```python
from build123d import *

# Parameters (mm, degrees)
F0_W     = 97.79
F0_H     = 57.15
F1_DEPTH = 14.7828
F2_W     = 38.1
F2_H     = 57.15
F3_DEPTH = 11.97483
F4_R     = 5
F6_DEPTH = 26.75863


with BuildPart() as f1:
    # F0 (on Front) → F1 (new body)
    with BuildSketch(Plane.XZ):
        with Locations((48.895, 28.575)):
            Rectangle(F0_W, F0_H)
    extrude(amount=F1_DEPTH)

    # F2 (on face) → F3 (join)
    with BuildSketch(Plane.XZ.offset(14.7828)):
        with Locations((48.895, 28.575)):
            Rectangle(F2_W, F2_H)
    extrude(amount=F3_DEPTH)

    # F4
    f4_edges = [f1.edges().sort_by_distance(p)[0] for p in [
        (0, -7.3914, 0),
        (29.845, -20.770215, 0),
        (67.945, -20.770215, 0),
        (97.79, -7.3914, 0),
        (97.79, -7.3914, 57.15),
        (67.945, -20.770215, 57.15),
        (29.845, -20.770215, 57.15),
        (0, -7.3914, 57.15),
    ]]
    fillet(f4_edges, radius=F4_R)

    # F5 (on face) → F6 (cut, through all)
    with BuildSketch(Plane(origin=(0, 0, 0), x_dir=(-1, 0, 0), z_dir=(0, 1, 0))):
        Polygon((-97.79, 58.0248906387), (-97.79, 28.575), (-92.79, 57.15), align=None)
        Polygon((-5, 57.15), (0, 28.575), (0, 58.0248906387), align=None)
    extrude(amount=-F6_DEPTH, mode=Mode.SUBTRACT)


solid = f1.part
```
Source: CAD feature listing. Evaluate the final solid. Frame: model axes, mm. A direction names the side the tool comes from. Coordinates: 2 decimals unless noted, no trailing zeros. Loops run counter-clockwise (first coordinate to the right, second up) from the corner with the lowest first, then second, coordinate; pieces in that order, holes last. Notation, with made-up numbers: (22, 81.5) -> (41, 81.5) arc R26 ccw to (41, 110.5) -> close; hole circle Ø1 at (29, 45.25). An arc over 180 degrees is marked (long way). One line per item, written item: value. Start each with the question number.
Q1. Contact query for flat-ended pins moving along their axis: P1, Ø10.5, axis at x = 85, z = 42.5, coming from the -Y side; P2, Ø3.5, axis at y = -20.5, z = 33, coming from the +X side (3 decimals); P3, Ø10, axis at y = -22, z = 49, coming from the -X side (3 decimals). Output: stop coordinate, or through.
Q2. Set-up query: faces 1 (the face through (31.349, -20.854, 55.724)), 2 (the face through (31.349, -20.854, 1.426)), 3 (the face through (29.845, -21, 28)), 4 (the face through (66.441, -20.854, 55.724)). Return all of +Z, -Z, +X, -X, +Y, -Y with unobstructed straight access to the full face (end or side cutting, diameter ignored); none if empty.
Q3. Section query B-B, the plane z = 19.5. Return the cut outline in (x, y) (3 decimals), and give its area (3 significant figures).
Q4. Section query A-A, the plane y = -19. Return the cut outline in (x, z) (3 decimals).
Q5. Line query: line 1 along X through (y, z) = (-21, 37) (3 decimals); line 2 along Y through (x, z) = (88, 9.5); line 3 along X through (y, z) = (-24.5, 53). Output: solid intervals per line, ascending.
Q6. Section query C-C, the plane x = 75. Return the cut outline in (y, z), and give its area (3 significant figures).
Results:
1. P1: y = -14.78
1. P2: x = 67.945
1. P3: x = 29.845
2. face 1: +Z, -X, -Y
2. face 2: -Z, -X, -Y
2. face 3: +Z, -Z, -X, -Y
2. face 4: +Z, +X, -Y
3. outline: (0, -14.783) -> (29.845, -14.783) -> (29.845, -26.758) -> (67.945, -26.758) -> (67.945, -14.783) -> (97.79, -14.783) -> (97.79, 0) -> (0, 0) -> close
3. area: 1,900 mm^2
4. outline: (29.845, 5) arc R5 ccw to (34.845, 0) -> (62.945, 0) arc R5 ccw to (67.945, 5) -> (67.945, 52.15) arc R5 ccw to (62.945, 57.15) -> (34.845, 57.15) arc R5 ccw to (29.845, 52.15) -> close
5. line 1: 29.845 to 67.945
5. line 2: -14.78 to 0
5. line 3: 29.92 to 67.87
6. outline: (-14.78, 0) -> (0, 0) -> (0, 57.15) -> (-14.78, 57.15) -> close
6. area: 845 mm^2
